For this review, take the finished solid that the model builds, in its own axes (mm). A direction names the side the tool comes from. Coordinates: 2 decimals unless noted, no trailing zeros. Write each loop counter-clockwise with the first axis right and the second up, starting at its lowest first coordinate (ties: lowest second). Pieces come first, ordered by that corner, then holes. Notation, with made-up numbers: M 8,76.5 L 38,76.5 A4 cw 38,81.5 Z; hole C 25,4.5 d1. An arc over 180 degrees is marked long. One line per question, with ' | ' between items.
from build123d import *

# Parameters (mm, degrees)
F1_W     = 9.4
F1_H     = 4
F2_DEPTH = 1.6
F4_W     = 15.8
F4_H     = 1.85
F4_W_2   = 12.1
F5_DEPTH = 3
F6_R     = 2.625
F7_DEPTH = 4.96
F8_W     = 20
F8_H     = 25.25
F9_DEPTH = 4


with BuildPart() as f2:
    # F1 (on offset) → F2 (new body)
    with BuildSketch(Plane.XY.offset(3)):
        Polygon((0.85, 12.875), (-10.25, 12.875), (-10.25, -12.875), (10.25, -12.875), (10.25, 12.875), align=None)
        with Locations((5.55, 14.875)):
            Rectangle(F1_W, F1_H)
    extrude(amount=F2_DEPTH)



with BuildPart() as f5:
    # F4 (on offset) → F5 (new body)
    with BuildSketch(Plane.XY):
        Polygon((10, -10.975), (10, 11.025), (9.05, 11.025), (-6.75, 11.025), (-10, 11.025), (-10, -10.975), (-5.8, -10.975), (6.3, -10.975), align=None)
        with Locations((1.15, 11.95)):
            Rectangle(F4_W, F4_H)
        with Locations((0.25, -11.9)):
            Rectangle(F4_W_2, F4_H)
    extrude(amount=F5_DEPTH)


with BuildPart() as f2_1:
    add(f2.part)

    add(f5.part)  # F7 merges F5
    # F6 (on face) → F7 (join)
    with BuildSketch(Plane(origin=(0, 12.875, 0), x_dir=(-1, 0, 0), z_dir=(0, 1, 0))):
        with Locations((-5.855308, 2.875)):
            Circle(F6_R)
    extrude(amount=F7_DEPTH)

    # F8 (on face) → F9 (join)
    with BuildSketch(Plane.XY.offset(4.6)):
        Rectangle(F8_W, F8_H)
    extrude(amount=F9_DEPTH)


solid = f2_1.part
1) We need section D-D on x = 5. State the section outline as (y, z) points (3 decimals), then the cut area to 3 significant figures.
Responses:
outline: M -12.875,3 L -12.825,3 L -12.825,0 L 12.875,0 L 12.875,0.393 L 17.835,0.393 L 17.835,5.357 L 12.875,5.357 L 12.875,4.6 L 12.625,4.6 L 12.625,8.6 L -12.625,8.6 L -12.625,4.6 L -12.875,4.6 Z | area: 244 mm^2
2) To check wall thickness, follow line 1 along X through (y, z) = (6, 7); line 2 along Y through (x, z) = (-4.5, 4.25) (3 decimals); line 3 along Y through (x, z) = (2.5, 1.5) (3 decimals). State the ranges of each line that lie inside material, in increasing order. Write a range as [from, to].
Responses:
line 1: [-10, 10] | line 2: [-12.875, 12.875] | line 3: [-12.825, 12.875]
3) We need section B-B on y = -5. State the section outline as (x, z) points, then the cut area to 3 significant figures.
Responses:
outline: M -10.25,3 L -10,3 L -10,0 L 10,0 L 10,3 L 10.25,3 L 10.25,4.6 L 10,4.6 L 10,8.6 L -10,8.6 L -10,4.6 L -10.25,4.6 Z | area: 173 mm^2
4) Insertion check: pin 1 Ø1.2 at (y, z) = (-1, 6) entering from +X; pin 2 Ø0.7 at (x, z) = (6, 5) entering from -Y (3 decimals); pin 3 Ø0.8 at (x, z) = (9.5, 2) entering from +Y (3 decimals). Each pin has a flat end and moves straight along its axis. Give the tip position at first contact, or say it passes through.
Responses:
pin 1: x = 10 | pin 2: y = -12.625 | pin 3: y = 11.025
5) We need section C-C on z = 1. State the section outline as (x, y) points (3 decimals).
Responses:
outline: M -10,-10.975 L -5.8,-10.975 L -5.8,-12.825 L 6.3,-12.825 L 6.3,-10.975 L 10,-10.975 L 10,11.025 L 9.05,11.025 L 9.05,12.875 L 7.692,12.875 L 7.692,17.835 L 4.018,17.835 L 4.018,12.875 L -6.75,12.875 L -6.75,11.025 L -10,11.025 Z
6) Machinability: for faces 4 (the flat face through (9.05, 12, 1)), 5 (the flat face through (-10, 0, 7)), 6 (the flat face through (-8, -10.975, 1)), 7 (the flat face through (10, 0, 1)), which of the approach directions +Z, -Z, +X, -X, +Y, -Y give a long, thin tool a straight path to every point of the face, cutting with its end or side? Answer none if there is none.
Responses:
face 4: -Z, +X, +Y | face 5: +Z, -X, +Y, -Y | face 6: -Z, -X, -Y | face 7: -Z, +X, +Y, -Y
7) The part is to be moulded in two halves that separate along Y. For faces 1 (the flat face through (6, 12.875, 5)), 2 (the flat face through (0, -12.825, 1)), 3 (the flat face through (10, 0, 7)), say which applies: +Y half, -Y half, draft (parallel to the pull), parting line (faces both ways), or undercut.
Responses:
face 1: undercut | face 2: -Y half | face 3: draft
8) We need section A-A on x = -2. State the section outline as (y, z) points (3 decimals), then the cut area to 3 significant figures.
Responses:
outline: M -12.875,3 L -12.825,3 L -12.825,0 L 12.875,0 L 12.875,4.6 L 12.625,4.6 L 12.625,8.6 L -12.625,8.6 L -12.625,4.6 L -12.875,4.6 Z | area: 219 mm^2
